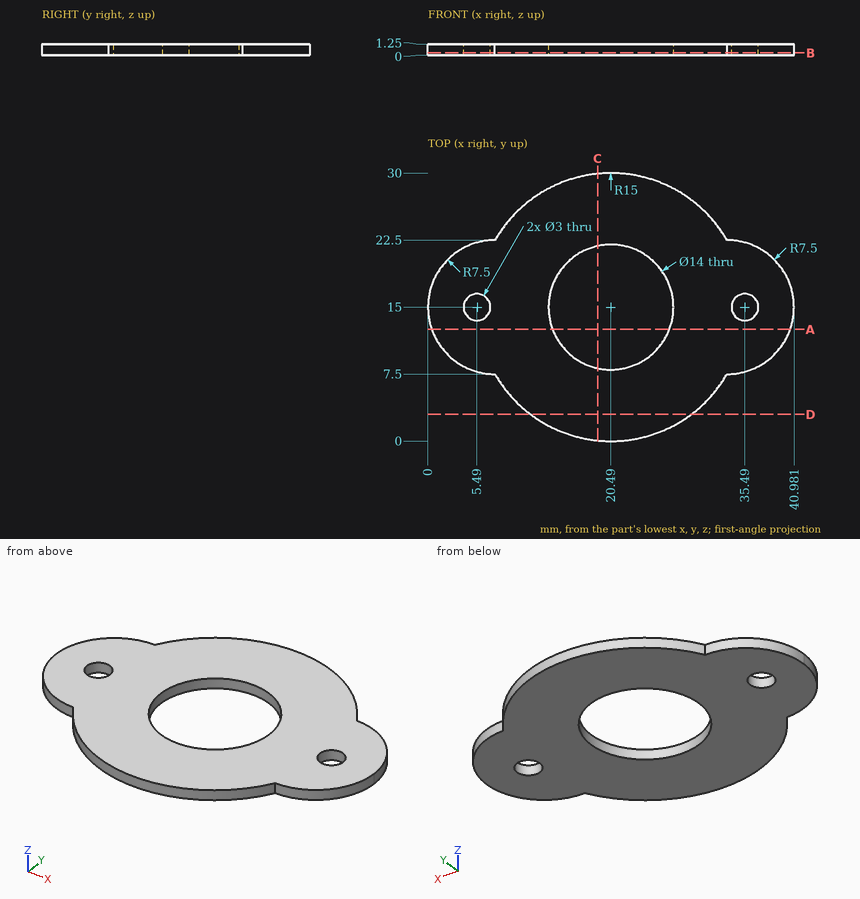
Design review of the part shown in the three views and the two pictorial views. Dimensions are in mm from the part's minimum x, y and z. Round coordinates to 2 decimals unless told otherwise and drop trailing zeros. Loops run counter-clockwise (first coordinate to the right, second up) from the corner with the lowest first, then second, coordinate; pieces in that order, holes last. Notation, with made-up numbers: (-16, 32.5) - (-1, 32.5) arc R8 ccw to (-1, 42.5) - close; hole circle Ø11 at (71, -16). An arc over 180 degrees is marked (long way). Use one line per item in the form item = value.
1) We need section D-D on y = 3. Write out the cut boundary in (x, z), then the cut area to 3 significant figures.
Solutions:
outline = (11.49, 0) - (29.49, 0) - (29.49, 1.25) - (11.49, 1.25) - close
area = 22.5 mm2
2) We need section C-C on x = 19. Write out the cut boundary in (y, z), then the cut area to 3 significant figures.
Solutions:
outline = (0.07, 0) - (8.16, 0) - (8.16, 1.25) - (0.07, 1.25) - close; (21.84, 0) - (29.93, 0) - (29.93, 1.25) - (21.84, 1.25) - close
area = 20.2 mm2
3) Wall thickness on probe 1 along Y at (x, z) = (18.5, 0.65); probe 2 along X at (y, z) = (10.5, 0.6); probe 3 along X at (y, z) = (20, 0.1): over which ranges is each line inside the solid? List them lowest first.
Solutions:
probe_1 = 0.13 to 8.29, 21.71 to 29.87
probe_2 = 1.5 to 15.13, 25.85 to 39.48
probe_3 = 1.91 to 15.59, 25.39 to 39.07
4) We need section B-B on z = 0.25. State how many separate pieces and enclosed holes the cut face has, then the cut area to 3 significant figures.
Solutions:
separate_pieces = 1
enclosed_holes = 3
area = 675 mm2
5) We need section A-A on y = 12.5. Write out the cut boundary in (x, z).
Solutions:
outline = (0.43, 0) - (13.95, 0) - (13.95, 1.25) - (0.43, 1.25) - close; (27.03, 0) - (40.55, 0) - (40.55, 1.25) - (27.03, 1.25) - close
